Verification items for the finished model (mm, model axes). A direction names the side the tool comes from. Give positions to 0.01 mm unless a question says otherwise; leave off trailing zeros. Write each loop counter-clockwise with the first axis right and the second up, starting at its lowest first coordinate (ties: lowest second). Pieces come first, ordered by that corner, then holes. Notation, with made-up numbers: (19, 18) -> (57, 18) arc R34 cw to (57, 50) -> close; hole circle Ø4 at (28, -3.5). An arc over 180 degrees is marked (long way). Answer as CSV lines item,"result". Start each with the question number.
1) Tool access check on faces 1 (the flat face through (0, 2, -5)), 2 (the flat face through (20, 2, -5)), 3 (the flat face through (10, 2, -10)), 4 (the flat face through (10, 2, 0)). Record the directions out of +Z, -Z, +X, -X, +Y, -Y that give a thin tool (end or side, any length) a straight path to the whole face; none if there is none.
2) Material ranges on L1, parallel to X at y = 0.5, z = -3.5; L2, parallel to Z at x = 17.5, y = 3; L3, parallel to Y at x = -1, z = -5.5, recorded low to high.
3) Sectioned sample at A-A on x = 4.25. Record the cut outline in (y, z), and give its area (3 significant figures).
4) Sectioned sample at C-C on y = 1. Record the cut outline in (x, z), and give its area (3 significant figures).
5) Sectioned sample at D-D on x = 21.25. Record the cut outline in (y, z), and give its area (3 significant figures).
6) Gauge pin test, flat ends, axial feed: pin 1 Ø2.5 at (x, y) = (7.5, 1.5) entering from -Z; pin 2 Ø2.5 at (x, y) = (6, 1.5) entering from +Z. Record the tip position at first contact, or that the pin passes through.
7) Sectioned sample at B-B on z = -9. Record the cut outline in (x, y).
```python
from build123d import *

# Parameters (mm, degrees)
SKETCH1_W           = 20
SKETCH1_H           = 10
BOSS_EXTRUDE1_DEPTH = 5
BOSS_EXTRUDE2_DEPTH = 2


with BuildPart() as part:
    # Sketch1 → Boss-Extrude1 (new body)
    with BuildSketch(Plane(origin=(0, 0, 0), x_dir=(1, 0, 0), z_dir=(0, 1, 0))):
        with Locations((10, 5)):
            Rectangle(SKETCH1_W, SKETCH1_H)
    extrude(amount=BOSS_EXTRUDE1_DEPTH)

    # Sketch2 → Boss-Extrude2 (add)
    with BuildSketch(Plane(origin=(0, 5, 0), x_dir=(1, 0, 0), z_dir=(0, 1, 0))):
        Polygon((-3, 13), (-3, 10), (-3, -3), (23, -3), (23, 13), align=None)
    extrude(amount=BOSS_EXTRUDE2_DEPTH)


solid = part.part
```
Ans:
1,face 1,"+Z, -Z, -X, -Y"
1,face 2,"+Z, -Z, +X, -Y"
1,face 3,"-Z, +X, -X, -Y"
1,face 4,"+Z, +X, -X, -Y"
2,L1,"x = 0 to 20"
2,L2,"z = -10 to 0"
2,L3,"y = 5 to 7"
3,outline,"(0, -10) -> (5, -10) -> (5, -13) -> (7, -13) -> (7, 3) -> (5, 3) -> (5, 0) -> (0, 0) -> close"
3,area,"82.0 mm²"
4,outline,"(0, -10) -> (20, -10) -> (20, 0) -> (0, 0) -> close"
4,area,"200 mm²"
5,outline,"(5, -13) -> (7, -13) -> (7, 3) -> (5, 3) -> close"
5,area,"32.0 mm²"
6,pin 1,"stops at z = -10"
6,pin 2,"stops at z = 0"
7,outline,"(-3, 5) -> (0, 5) -> (0, 0) -> (20, 0) -> (20, 5) -> (23, 5) -> (23, 7) -> (-3, 7) -> close"
